Check sheet for the modelled part. Datum: model origin and axes. Units: mm. A direction names the side the tool comes from. Give positions to 0.01 mm unless a question says otherwise; leave off trailing zeros. Loops run counter-clockwise (first coordinate to the right, second up) from the corner with the lowest first, then second, coordinate; pieces in that order, holes last. Notation, with made-up numbers: (46, -11.75) - (100, -11.75) arc R17 ccw to (100, 6.25) - close; hole circle Ø8 at (46, 29). An arc over 180 degrees is marked (long way). Answer in a Markdown table with one row per item. Add a question column.
(1) Sectioned sample at A-A on y = 6. Enter the section's corners in (x, z) (3 decimals).
(2) Thickness scan on L1, parallel to Z at x = 1.75, y = 90; L2, parallel to Z at x = 2.75, y = 86.5; L3, parallel to X at y = 56.5, z = -2.5. Record the ranges inside material, lowest first.
(3) Draft check along Y on faces 5 (the face through (2, 92.456, -2)), 6 (the face through (-1.7, 34.544, 2.9)), 7 (the face through (-1.62, 91.94, -2.12)), 8 (the face through (-1.93, 62.59, -2.52)). Enter one of: released by +Y, released by -Y, zero draft, split by the parting line, or undercut.
(4) Go/stop test with flat-tipped pins: P1, Ø3, axis at y = 12, z = 2.5, coming from the -X side; P2, Ø2, axis at y = 74, z = -0.5, coming from the -X side (3 decimals). Record where each tip stops, or that it passes through.
(5) Set-up check for faces 1 (the face through (1.7, 0, -2.9)), 2 (the face through (-1.7, 0, 2.9)), 3 (the face through (1.7, 34.544, -2.9)), 4 (the face through (-1.7, 0, -2.9)): record each of +Z, -Z, +X, -X, +Y, -Y from which the full face is reachable in a straight line by a thin tool's end or side.
(6) Sectioned sample at B-B on y = 55. Enter the section's corners in (x, z) (3 decimals), then the cut area to 3 significant figures.
from build123d import *

# Parameters (mm, degrees)
BOSS_EXTRUDE1_DEPTH = 34.544
SKETCH2_R           = 3.175
BOSS_EXTRUDE2_DEPTH = 56.896
SKETCH3_R           = 2.667
BOSS_EXTRUDE3_DEPTH = 1.016
SKETCH4_R           = 3.175
BOSS_EXTRUDE4_DEPTH = 2.286
BOSS_EXTRUDE5_START = 9.906
SKETCH5_R           = 3.175
BOSS_EXTRUDE5_DEPTH = 9.906


with BuildPart() as part:
    # Sketch1 → Boss-Extrude1 (new body)
    with BuildSketch(Plane(origin=(0, 0, 0), x_dir=(1, 0, 0), z_dir=(0, 1, 0))):
        Polygon((1.833087105, 3.175), (-1.833087105, 3.175), (-3.666174209, 0), (-1.833087105, -3.175), (1.833087105, -3.175), (3.666174209, 0), align=None)
    extrude(amount=BOSS_EXTRUDE1_DEPTH)

    # Sketch2 → Boss-Extrude2 (add)
    with BuildSketch(Plane(origin=(0, 34.544, 0), x_dir=(1, 0, 0), z_dir=(0, 1, 0))):
        with Locations(Location((0, 0, 0), (0, 0, 270))):
            Circle(SKETCH2_R)
    extrude(amount=BOSS_EXTRUDE2_DEPTH)

    # Sketch3 → Boss-Extrude3 (add)
    with BuildSketch(Plane(origin=(0, 91.44, 0), x_dir=(1, 0, 0), z_dir=(0, 1, 0))):
        with Locations(Location((0, 0, 0), (0, 0, 270))):
            Circle(SKETCH3_R)
    extrude(amount=BOSS_EXTRUDE3_DEPTH)

    # Sketch4 → Boss-Extrude4 (add)
    with BuildSketch(Plane(origin=(0, 92.456, 0), x_dir=(1, 0, 0), z_dir=(0, 1, 0))):
        with Locations(Location((0, 0, 0), (0, 0, 270))):
            Circle(SKETCH4_R)
    extrude(amount=BOSS_EXTRUDE4_DEPTH)

    # Sketch5 → Boss-Extrude5 (add)
    with BuildSketch(Plane.XZ.offset(BOSS_EXTRUDE5_START)):
        with Locations(Location((0, 0, 0), (0, 0, 90))):
            Circle(SKETCH5_R)
    extrude(amount=-BOSS_EXTRUDE5_DEPTH)


solid = part.part
Reply:
| question | item | result |
|---|---|---|
| 1 | outline | (-3.666, 0) - (-1.833, -3.175) - (1.833, -3.175) - (3.666, 0) - (1.833, 3.175) - (-1.833, 3.175) - close |
| 2 | L1 | -2.65 to 2.65 |
| 2 | L2 | -1.59 to 1.59 |
| 2 | L3 | -1.96 to 1.96 |
| 3 | face 5 | undercut |
| 3 | face 6 | released by +Y |
| 3 | face 7 | undercut |
| 3 | face 8 | zero draft |
| 4 | P1 | x = -3.09 |
| 4 | P2 | x = -3.175 |
| 5 | face 1 | -Z, +X, -Y |
| 5 | face 2 | +Z, -X, -Y |
| 5 | face 3 | -Z, +X, +Y |
| 5 | face 4 | -Z, -X, -Y |
| 6 | outline | circle Ø6.35 at (0, 0) |
| 6 | area | 31.7 mm^2 |
